Answer from the drawing. Dimensions are ordinates in mm from the lowest x, y and z of the part. Coordinates: 2 decimals unless noted, no trailing zeros. Order: outer loops, then holes, each group sorted by start corner. A loop starts at its lowest first (then second) coordinate and runs counter-clockwise, first axis right, second up. Notation, with made-up numbers: (-18.5, -31) - (0.5, -31) arc R17 ccw to (0.5, -13) - close; hole circle Ø1 at (35.5, 18). An arc over 180 degrees is marked (long way). Use a Markdown table: item, result. Add a question column.
Item 1: The part is cut by section D-D, the plane z = 0.7. Give the vertices of the cut face in (x, y) (1 decimal), then the cut area to 3 significant figures.
Item 2: The part is cut by section A-A, the plane z = 1.9. Give the vertices of the cut face in (x, y) (1 decimal), then the cut area to 3 significant figures.
Item 3: A flat-ended cylindrical pin translates along its axis: P1, Ø1, axis at y = 5, z = 1, coming from the +X side. Find the tip coordinate at first contact, or state that the pin passes through.
Item 4: The part is cut by section C-C, the plane x = 3.6. Give the vertices of the cut face in (y, z) (1 decimal).
Item 5: Find the intervals of material crossed by line 1 along Z through (x, y) = (2, 2.4) (1 decimal); line 2 along X through (y, z) = (4.7, 1.5) (1 decimal); line 3 along Z through (x, y) = (1.95, 4.6) (1 decimal), in increasing order.
Item 6: The mould has two halves that part along Z. Classify the marked faces 1, 2, 3 and 4: released by +Z, released by -Z, zero draft, split by the parting line, or undercut.
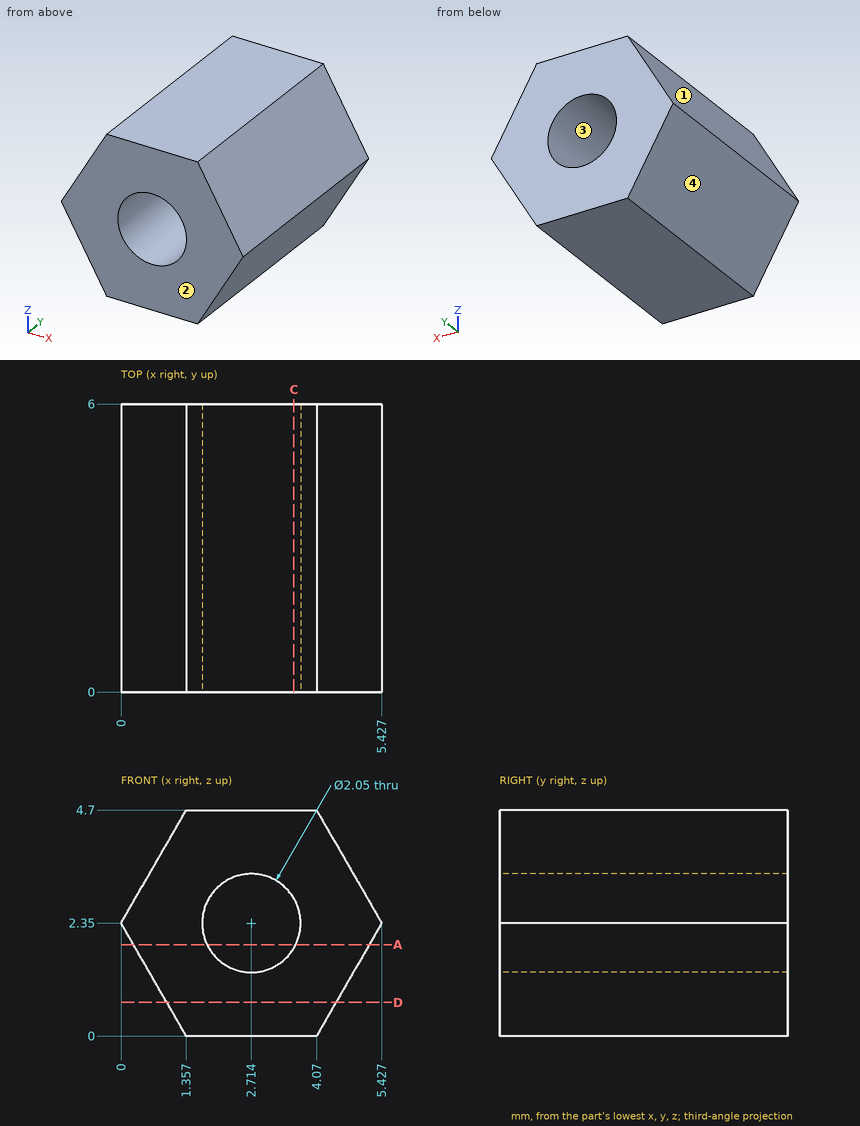
Solution:
| question | item | result |
|---|---|---|
| 1 | outline | (1, 0) - (4.5, 0) - (4.5, 6) - (1, 6) - close |
| 1 | area | 21.1 mm2 |
| 2 | outline | (0.3, 0) - (1.8, 0) - (1.8, 6) - (0.3, 6) - close; (3.6, 0) - (5.2, 0) - (5.2, 6) - (3.6, 6) - close |
| 2 | area | 18.4 mm2 |
| 3 | P1 | stops at x = 4.94 |
| 4 | outline | (0, 0) - (6, 0) - (6, 1.8) - (0, 1.8) - close; (0, 2.9) - (6, 2.9) - (6, 4.7) - (0, 4.7) - close |
| 5 | line 1 | z = 0 to 1.6, 3.1 to 4.7 |
| 5 | line 2 | x = 0.5 to 2.1, 3.3 to 4.9 |
| 5 | line 3 | z = 0 to 1.7, 3 to 4.7 |
| 6 | face 1 | released by +Z |
| 6 | face 2 | zero draft |
| 6 | face 3 | undercut |
| 6 | face 4 | released by -Z |
